```python
from build123d import *

# Parameters (mm, degrees)
BOSS_EXTRUDE1_DEPTH = 50
SKETCH2_W           = 56
SKETCH2_H           = 91
CUT_EXTRUDE1_DEPTH  = 65.651656333
CUT_EXTRUDE2_START  = -1
SKETCH3_W           = 60
SKETCH3_H           = 95
CUT_EXTRUDE2_DEPTH  = 2.2


with BuildPart() as part:
    # Sketch1 → Boss-Extrude1 (new, symmetric)
    with BuildSketch(Plane(origin=(0, 0, 0), x_dir=(1, 0, 0), z_dir=(0, 1, 0))):
        with BuildLine():
            Line((-36.796835842, -43.531515848), (-32.9234847, -38.949251022))
            Line((-32.9234847, -38.949251022), (32.9234847, -38.949251022))
            Line((32.9234847, -38.949251022), (36.796835842, -43.531515848))
            ThreePointArc((36.796835842, -43.531515848), (0, -57), (-36.796835842, -43.531515848))
        make_face()
    extrude(amount=BOSS_EXTRUDE1_DEPTH, both=True)

    # Sketch2 → Cut-Extrude1 (cut, through all)
    with BuildSketch(Plane(origin=(0, 0, 38.949251022), x_dir=(-1, 0, 0), z_dir=(0, 0, -1))):
        Rectangle(SKETCH2_W, SKETCH2_H)
    extrude(amount=-CUT_EXTRUDE1_DEPTH, mode=Mode.SUBTRACT)

    # Sketch3 → Cut-Extrude2 (cut)
    with BuildSketch(Plane(origin=(0, 0, 38.949251022), x_dir=(-1, 0, 0), z_dir=(0, 0, -1)).offset(CUT_EXTRUDE2_START)):
        Rectangle(SKETCH3_W, SKETCH3_H)
    extrude(amount=-CUT_EXTRUDE2_DEPTH, mode=Mode.SUBTRACT)


solid = part.part
```
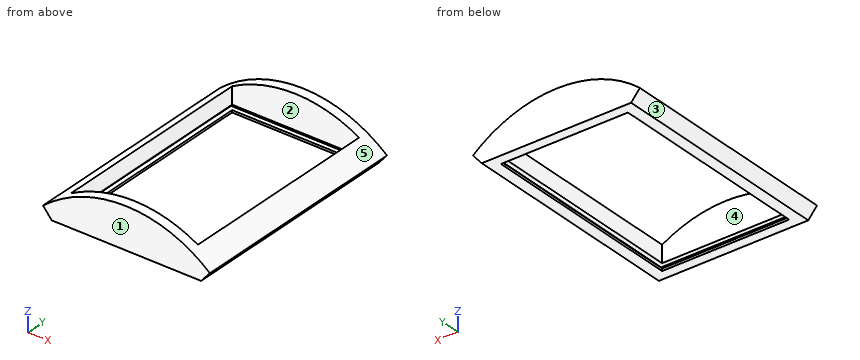
Model file for the job. Use its own axes, mm. Face numbers are marked on the shaded views. A direction names the side the tool comes from. Coordinates: 2 decimals unless noted, no trailing zeros. Order: outer loops, then holes, each group sorted by start corner. A loop starts at its lowest first (then second) coordinate and runs counter-clockwise, first axis right, second up. Notation, with made-up numbers: M 0.5,40 L 39.5,40 A10 cw 39.5,44 Z; hole C 70,34 d8. An arc over 180 degrees is marked long. Answer as CSV lines item,"result".
(1) Band-saw the part on B-B, the plane y = 38.5. List the corners of the cut face in (x, z), then the cut area to 3 significant figures.
Geometry says:
outline,"M -36.8,43.53 L -32.92,38.95 L -28,38.95 L -28,39.95 L -30,39.95 L -30,42.15 L -28,42.15 L -28,49.65 A57 ccw Z; M 28,38.95 L 32.92,38.95 L 36.8,43.53 A57 ccw 28,49.65 L 28,42.15 L 30,42.15 L 30,39.95 L 28,39.95 Z"
area,"111 mm2"
(2) 3-axis set-ups, long thin cutter, end or side, ignore diameter. For the marked faces 4 and 5: which of +Z, -Z, +X, -X, +Y, -Y reach the whole face in a straight line?
Geometry says:
face 4,"+Z, -Z"
face 5,"+Z, +Y, -Y"
(3) Band-saw the part on A-A, the plane x = -24.5. List the corners of the cut face in (y, z).
Geometry says:
outline,"M -50,38.95 L -45.5,38.95 L -45.5,39.95 L -47.5,39.95 L -47.5,42.15 L -45.5,42.15 L -45.5,51.47 L -50,51.47 Z; M 45.5,38.95 L 50,38.95 L 50,51.47 L 45.5,51.47 L 45.5,42.15 L 47.5,42.15 L 47.5,39.95 L 45.5,39.95 Z"
(4) Band-saw the part on D-D, the plane z = 44.75. List the corners of the cut face in (x, y).
Geometry says:
outline,"M -35.3,-50 L 35.3,-50 L 35.3,50 L -35.3,50 Z; hole M -28,-45.5 L 28,-45.5 L 28,45.5 L -28,45.5 Z"
(5) Band-saw the part on C-C, the plane z = 54.75. List the corners of the cut face in (x, y), then the cut area to 3 significant figures.
Geometry says:
outline,"M -15.86,-50 L 15.86,-50 L 15.86,-45.5 L -15.86,-45.5 Z; M -15.86,45.5 L 15.86,45.5 L 15.86,50 L -15.86,50 Z"
area,"285 mm2"
(6) Wall check: line 1 along Y through (x, z) = (3, 43); line 2 along Y through (x, z) = (-3, 41); line 3 along Z through (x, y) = (-31.5, 36.5). Give the ranges that are in metal, low to high.
Geometry says:
line 1,"y = -50 to -45.5, 45.5 to 50"
line 2,"y = -50 to -47.5, 47.5 to 50"
line 3,"z = 38.95 to 47.51"
(7) Pull direction Y, two halves, no side cores. Call the marked faces 1, 2 and 3: +Y half, -Y half, draft (parallel to the pull), parting line (faces both ways), or undercut.
Geometry says:
face 1,"-Y half"
face 2,"undercut"
face 3,"draft"
(8) Flat gauge pins, fed straight in: pin 1 (2.5 mm diameter, centred on y = -12.5, z = 41.5, fed in from -X); pin 2 (2.5 mm diameter, centred on y = 15, z = 41, fed in from +X); pin 3 (0.8 mm diameter, centred on y = -8.5, z = 39.5, fed in from +X). Where does each tip first touch, or does it go through?
Geometry says:
pin 1,"stops at x = -36.14"
pin 2,"stops at x = 35.71"
pin 3,"stops at x = 33.73"
